Model file for the job. Use its own axes, mm. A direction names the side the tool comes from. Coordinates: 2 decimals unless noted, no trailing zeros. Order: outer loops, then holes, each group sorted by start corner. A loop starts at its lowest first (then second) coordinate and runs counter-clockwise, first axis right, second up. Notation, with made-up numbers: (6.5, 88) -> (25.5, 88) arc R30 cw to (25.5, 114) -> close; hole circle Ø9 at (20, 25). An arc over 180 degrees is marked (long way). Return JSON: item names as keys, results as strings. Group by question number.
1) Probe line 1 (X direction, y = 5.35, z = 0); line 2 (Z direction, x = 9.5, y = 0); line 3 (X direction, y = 2.5, z = -9.5). List the from-to ranges inside material, lowest first.
2) Which spindle directions (+Z, -Z, +X, -X, +Y, -Y) get a long thin tool onto all of the face, cutting with end or side? Do faces 1 (the flat face through (7, 0, -12)), 2 (the flat face through (14.96, 5.31, -8.46)), 3 (the flat face through (5.51, 11.74, -0.87)). Say none if no direction does.
3) Flat gauge pins, fed straight in: pin 1 (1.5 mm diameter, centred on x = 3, y = -3.5, fed in from +Z); pin 2 (1.6 mm diameter, centred on x = 6, z = 0, fed in from +Y); pin 3 (1.9 mm diameter, centred on x = 6, y = 0, fed in from -Z). Where does each tip first touch, or does it go through?
4) Pull direction Y, two halves, no side cores. Call faces 4 (the cylindrical face through (14.958, 10.147, 4.499)), 5 (the flat face through (6.49, 11.74, 0.87)), 6 (the flat face through (6, 11, 0)): +Y half, -Y half, draft (parallel to the pull), parting line (faces both ways), or undercut.
5) Cut at C-C (x = 9). Write the cut outline in (y, z), and give its area (3 significant figures).
Autodesk Inventor part; units mm, degrees
ref_plane "left_XY" through (12, 0, 0) normal (1, 0, 0) x (0, 0, -1)
ref_plane "left_YZ" through (12, 0, 0) normal (0, 0, -1) x (0, 1, 0)
ref_plane "left_ZX" through (12, 0, 0) normal (0, 1, 0) x (1, 0, 0)
sketch "Sketch_1" plane through (0, 0, 0) normal (0, 0, 1) x (1, 0, 0)
  line L0 (18, 0) -> (0, 0)
  line L1 (0, 0) -> (0, 12)
  line L2 (0, 12) -> (0.5, 12.5)
  line L3 (0.5, 12.5) -> (17.5, 12.5)
  line L4 (17.5, 12.5) -> (18, 12)
  line L5 (18, 12) -> (18, 0)
  line L6 (18, 0) -> (0, 0)
revolve "Revolution1" add sketch "Sketch_1" angle 360 about axis through (18, 0, 0) along (1, 0, 0)
sketch "Sketch_2" plane through (12, 0, 0) normal (1, 0, 0) x (0, 0, -1)
  line L0 (-10.681, 3.0208) -> (-8.764, 1.4122)
  arc A0 (-8.764, -1.4122) -> (-8.764, 1.4122) centre (-10.005, 0) ccw
  line L1 (-8.764, -1.4122) -> (-10.5287, -3.5153)
  arc A1 (-10.5287, -3.5153) -> (-9.6887, -5.4166) centre (0, 0) ccw
  line L2 (-9.6887, -5.4166) -> (-7.1956, -5.1985)
  arc A2 (-5.1985, -7.1956) -> (-7.1956, -5.1985) centre (-7.0746, -7.0746) ccw
  line L3 (-5.1985, -7.1956) -> (-4.9592, -9.9306)
  arc A3 (-4.9592, -9.9306) -> (-3.0208, -10.681) centre (0, 0) ccw
  line L4 (-3.0208, -10.681) -> (-1.4122, -8.764)
  arc A4 (1.4122, -8.764) -> (-1.4122, -8.764) centre (0, -10.005) ccw
  line L5 (1.4122, -8.764) -> (3.5153, -10.5287)
  arc A5 (3.5153, -10.5287) -> (5.4166, -9.6887) centre (0, 0) ccw
  line L6 (5.4166, -9.6887) -> (5.1985, -7.1956)
  arc A6 (7.1956, -5.1985) -> (5.1985, -7.1956) centre (7.0746, -7.0746) ccw
  line L7 (7.1956, -5.1985) -> (9.9306, -4.9592)
  arc A7 (9.9306, -4.9592) -> (10.681, -3.0208) centre (0, 0) ccw
  line L8 (10.681, -3.0208) -> (8.764, -1.4122)
  arc A8 (8.764, 1.4122) -> (8.764, -1.4122) centre (10.005, 0) ccw
  line L9 (8.764, 1.4122) -> (10.5287, 3.5153)
  arc A9 (10.5287, 3.5153) -> (9.6887, 5.4166) centre (0, 0) ccw
  line L10 (9.6887, 5.4166) -> (7.1956, 5.1985)
  arc A10 (5.1985, 7.1956) -> (7.1956, 5.1985) centre (7.0746, 7.0746) ccw
  line L11 (5.1985, 7.1956) -> (4.9592, 9.9306)
  arc A11 (4.9592, 9.9306) -> (3.0208, 10.681) centre (0, 0) ccw
  line L12 (3.0208, 10.681) -> (1.4122, 8.764)
  arc A12 (-1.4122, 8.764) -> (1.4122, 8.764) centre (0, 10.005) ccw
  line L13 (-1.4122, 8.764) -> (-3.5153, 10.5287)
  arc A13 (-3.5153, 10.5287) -> (-5.4166, 9.6887) centre (0, 0) ccw
  line L14 (-5.4166, 9.6887) -> (-5.1985, 7.1956)
  arc A14 (-7.1956, 5.1985) -> (-5.1985, 7.1956) centre (-7.0746, 7.0746) ccw
  line L15 (-7.1956, 5.1985) -> (-9.9306, 4.9592)
  arc A15 (-9.9306, 4.9592) -> (-10.681, 3.0208) centre (0, 0) ccw
extrude "Extrusion1" cut sketch "Sketch_2" along normal blind 6
sketch "Sketch_3" plane through (0, 0, 0) normal (1, 0, 0) x (0, 1, 0)
  circle A0 centre (0, 0) radius 3
extrude "Extrusion2" cut sketch "Sketch_3" along normal mid plane 34
sketch "Sketch_4" plane through (0, 0, 0) normal (0, 0, 1) x (1, 0, 0)
  line L0 (6, 0) -> (6, 12.5)
  line L1 (6, 12.5) -> (8, 12.5)
  line L2 (8, 12.5) -> (7.6211, 12.1211)
  line L3 (7.6211, 12.1211) -> (7.6211, 0.3789)
  line L4 (7.6211, 0.3789) -> (8, 0)
  line L5 (8, 0) -> (6, 0)
  line L6 (6, 0) -> (6, 12.5)
revolve "Revolution2" cut sketch "Sketch_4" angle 360 about axis through (6, 0, 0) along (0, -1, 0)
sketch "Sketch_6" plane through (0, 0, 0) normal (0, 1, 0) x (-1, 0, 0)
  line L0 (-6, 0) -> (-6, -12.5)
  line L1 (-6, -12.5) -> (-8, -12.5)
  line L2 (-8, -12.5) -> (-7.6211, -12.1211)
  line L3 (-7.6211, -12.1211) -> (-7.6211, -0.3789)
  line L4 (-7.6211, -0.3789) -> (-8, 0)
  line L5 (-8, 0) -> (-6, 0)
  line L6 (-6, 0) -> (-6, -12.5)
revolve "Revolution3" cut sketch "Sketch_6" angle 360 about axis through (6, 0, 0) along (0, 0, 1)
sketch "Sketch_8" plane through (0, 0, 0) normal (0, 0, 1) x (1, 0, 0)
  line L0 (6, 6.5) -> (6, 12.5)
  line L1 (6, 12.5) -> (7.6211, 12.5)
  line L2 (7.6211, 12.5) -> (8, 12.1211)
  line L3 (8, 12.1211) -> (8, 6.8789)
  line L4 (8, 6.8789) -> (7.6211, 6.5)
  line L5 (7.6211, 6.5) -> (6, 6.5)
  line L6 (6, 6.5) -> (6, 12.5)
revolve "Revolution4" add sketch "Sketch_8" angle 360 about axis through (6, 6.5, 0) along (0, -1, 0)
sketch "Sketch_5" plane through (0, 11, 0) normal (0, 1, 0) x (1, 0, 0)
  line L0 (5, -0.5774) -> (6, -1.1547)
  line L1 (6, -1.1547) -> (7, -0.5774)
  line L2 (7, -0.5774) -> (7, 0.5774)
  line L3 (7, 0.5774) -> (6, 1.1547)
  line L4 (6, 1.1547) -> (5, 0.5774)
  line L5 (5, 0.5774) -> (5, -0.5774)
extrude "Extrusion3" cut sketch "Sketch_5" along normal blind 1.5
sketch "Sketch_7" plane through (0, 0, 0) normal (0, 1, 0) x (-1, 0, 0)
  line L0 (-6, -6.5) -> (-6, -12.5)
  line L1 (-6, -12.5) -> (-7.6211, -12.5)
  line L2 (-7.6211, -12.5) -> (-8, -12.1211)
  line L3 (-8, -12.1211) -> (-8, -6.8789)
  line L4 (-8, -6.8789) -> (-7.6211, -6.5)
  line L5 (-7.6211, -6.5) -> (-6, -6.5)
  line L6 (-6, -6.5) -> (-6, -12.5)
revolve "Revolution5" add sketch "Sketch_7" angle 360 about axis through (6, 0, -6.5) along (0, 0, 1)
sketch "Sketch_9" plane through (0, 0, -12.5) normal (0, 0, 1) x (1, 0, 0)
  line L0 (5, -0.5774) -> (6, -1.1547)
  line L1 (6, -1.1547) -> (7, -0.5774)
  line L2 (7, -0.5774) -> (7, 0.5774)
  line L3 (7, 0.5774) -> (6, 1.1547)
  line L4 (6, 1.1547) -> (5, 0.5774)
  line L5 (5, 0.5774) -> (5, -0.5774)
extrude "Extrusion4" cut sketch "Sketch_9" along normal blind 1.5
ref_plane "left_XY" through (12, 0, 0) normal (1, 0, 0) x (0, 0, -1)
ref_plane "left_YZ" through (12, 0, 0) normal (0, 0, -1) x (0, 1, 0)
ref_plane "left_ZX" through (12, 0, 0) normal (0, 1, 0) x (1, 0, 0)
ref_plane "left_dummy_XY" through (0, 0, 0) normal (1, 0, 0) x (0, 0, -1)
ref_plane "left_dummy_YZ" through (0, 0, 0) normal (0, 0, -1) x (0, 1, 0)
ref_plane "left_dummy_ZX" through (0, 0, 0) normal (0, 1, 0) x (1, 0, 0)
properties part number "MSF-25 - 6-8 Casing 1"
Answers below:
{
 "1": {"line 1": "x = 0 to 4.38, 7.62 to 12", "line 2": "z = -12.5 to -3, 3 to 12.5", "line 3": "x = 0 to 12"},
 "2": {"face 1": "-Z", "face 2": "+X", "face 3": "+Y"},
 "3": {"pin 1": "stops at z = 12.19", "pin 2": "stops at y = 11", "pin 3": "stops at z = -11"},
 "4": {"face 4": "undercut", "face 5": "draft", "face 6": "+Y half"},
 "5": {"outline": "circle Ø25 at (0, 0); hole circle Ø6 at (0, 0)", "area": "463 mm^2"}
}
